Could you check a few things on this model? Use its own coordinates, in mm. Coordinates: 2 decimals unless noted, no trailing zeros. Write each loop counter-clockwise with the first axis right and the second up, starting at its lowest first coordinate (ties: lowest second). Pieces come first, ordered by that corner, then holes. Notation, with made-up numbers: (54.5, 80.25) - (105.5, 80.25) arc R15 ccw to (105.5, 98.25) - close; hole circle Ø3 at (-26, 31.5). An arc over 180 degrees is marked (long way). Answer as a JSON object with one key per item and string values. Group by question number.
1) Please list where these lines run through material, in increasing order: line 1 along Y through (x, z) = (31.75, 5); line 2 along Y through (x, z) = (6.35, 4); line 3 along X through (y, z) = (-44.5, 1.75) (3 decimals).
2) If we section it at D-D (x = 96.5): Write out the boundary of the cut face in (y, z) (3 decimals), plus the area to 3 significant figures.
3) We'd pull the mould along Y, two halves only. Please class faces 1 (the cylindrical face through (5.89, -40.91, 3.13)), 2 (the flat face through (66, -29, 6.35)), 3 (the flat face through (116, -76.2, 3)): released by +Y, released by -Y, zero draft, split by the parting line, or undercut.
4) If we section it at B-B (y = -6.35): Write out the boundary of the cut face in (x, z) (3 decimals).
5) If we section it at C-C (y = -66): Write out the boundary of the cut face in (x, z) (3 decimals).
6) If we section it at A-A (x = 6.35): Write out the boundary of the cut face in (y, z), plus the area to 3 significant figures.
7) Will this pin go through, and if not, where does the flat tip stop? pin 1 Ø5.5 at (x, y) = (6.35, -6.35) entering from -Z.
```python
from build123d import *

# Parameters (mm, degrees)
F0_R        = 3.5687
F1_DEPTH    = 6.35
F2_T1_DEPTH = 67.1301869736


# Not quite as in the source:
# - a fillet or chamfer that OpenCascade refuses, or shapes differently, is made with other operations: its cross-section is extruded or revolved along the edge and cut away or added


with BuildPart() as f1:
    # F0 (on Top) → F1 (new body)
    with BuildSketch(Plane.XY):
        Polygon((130.175, 0), (0, 0), (0, -50.8), (101.6, -76.2), (130.175, -76.2), align=None)
        with Locations((6.35, -44.45)):
            Circle(F0_R, mode=Mode.SUBTRACT)
        with Locations((31.75, -44.45)):
            Circle(F0_R, mode=Mode.SUBTRACT)
        with Locations((6.35, -6.35)):
            Circle(F0_R, mode=Mode.SUBTRACT)
        with Locations((31.75, -6.35)):
            Circle(F0_R, mode=Mode.SUBTRACT)
    extrude(amount=F1_DEPTH)

    # F2: chamfer of 3.175 on 1 edges, made by hand

    # F2_s2 → F2_t1 (cut)
    with BuildSketch(Plane.XZ.offset(-8.1650934868)):
        Polygon((0, 3.175), (3.175, 6.35), (0, 6.35), align=None)
    extrude(amount=F2_T1_DEPTH, mode=Mode.SUBTRACT)


solid = f1.part
```
Here are the results:
{
 "1": {"line 1": "y = -58.74 to -48.02, -40.88 to -9.92, -2.78 to 0", "line 2": "y = -52.39 to -48.02, -40.88 to -9.92, -2.78 to 0", "line 3": "x = 0 to 2.782, 9.918 to 28.182, 35.318 to 130.175"},
 "2": {"outline": "(-74.925, 0) - (0, 0) - (0, 6.35) - (-74.925, 6.35) - close", "area": "476 mm²"},
 "3": {"face 1": "undercut", "face 2": "zero draft", "face 3": "released by -Y"},
 "4": {"outline": "(0, 0) - (2.781, 0) - (2.781, 5.956) - (0, 3.175) - close; (9.919, 0) - (28.181, 0) - (28.181, 6.35) - (9.919, 6.35) - close; (35.319, 0) - (130.175, 0) - (130.175, 6.35) - (35.319, 6.35) - close"},
 "5": {"outline": "(60.8, 0) - (130.175, 0) - (130.175, 6.35) - (60.8, 6.35) - close"},
 "6": {"outline": "(-52.39, 0) - (-48.02, 0) - (-48.02, 6.35) - (-52.39, 6.35) - close; (-40.88, 0) - (-9.92, 0) - (-9.92, 6.35) - (-40.88, 6.35) - close; (-2.78, 0) - (0, 0) - (0, 6.35) - (-2.78, 6.35) - close", "area": "242 mm²"},
 "7": {"pin 1": "passes through"}
}
